from build123d import *

# Parameters (mm, degrees)
F0_R     = 25.4
F1_DEPTH = 12.7
F2_R     = 8.6995
F3_DEPTH = 25.4
F4_W     = 19.947653
F4_H     = 8.920466
F5_DEPTH = 6.35
F6_SIZE  = 0.635


with BuildPart() as f1:
    # F0 (on Top) → F1 (new body)
    with BuildSketch(Plane.XY):
        Circle(F0_R)
    extrude(amount=F1_DEPTH)

    # F2 (on face) → F3 (cut)
    with BuildSketch(Plane.XY.offset(12.7)):
        Circle(F2_R)
    extrude(amount=-F3_DEPTH, mode=Mode.SUBTRACT)

    # F4 (on face) → F5 (cut)
    with BuildSketch(Plane.XY.offset(12.7)):
        with Locations((-17.442937, 0)):
            Rectangle(F4_W, F4_H)
    extrude(amount=-F5_DEPTH, mode=Mode.SUBTRACT)

    # F6
    f6_edges = [f1.edges().sort_by_distance(p)[0] for p in [
        (-8.6995, 0, 0),
    ]]
    chamfer(f6_edges, length=F6_SIZE)


solid = f1.part
Build history of the part. All positions in model axes, mm. A direction names the side the tool comes from. Round coordinates to 2 decimals unless told otherwise and drop trailing zeros. Write each loop counter-clockwise with the first axis right and the second up, starting at its lowest first coordinate (ties: lowest second). Pieces come first, ordered by that corner, then holes. Notation, with made-up numbers: M 77.5,14 L 130.5,14 A21 ccw 130.5,40 Z; hole C 46,21.25 d7. An arc over 180 degrees is marked long. Answer in a Markdown table with one row per item.
1. Which spindle directions (+Z, -Z, +X, -X, +Y, -Y) get a long thin tool onto all of the face, cutting with end or side? Do faces 1 (the face through (11, 0, 12.7)), 2 (the face through (-17, 0, 6.35)). Say none if no direction does.
Geometry check:
| item | result |
|---|---|
| face 1 | +Z, +X, -X, +Y, -Y |
| face 2 | +Z, -X |
2. Saw through at D-D (y = 19.5). List the corners of the cut face in (x, z).
Geometry check:
| item | result |
|---|---|
| outline | M -16.28,0 L 16.28,0 L 16.28,12.7 L -16.28,12.7 Z |
3. Probe L1, parallel to Y at x = 0, z = 9.25; L2, parallel to Y at x = -2, z = 5.75; L3, parallel to X at y = -4, z = 6. List the from-to ranges inside material, lowest first. Write a range as [from, to].
Geometry check:
| item | result |
|---|---|
| L1 | [-25.4, -8.7], [8.7, 25.4] |
| L2 | [-25.32, -8.47], [8.47, 25.32] |
| L3 | [-25.08, -7.73], [7.73, 25.08] |
4. Saw through at B-B (x = -19.5). List the corners of the cut face in (y, z).
Geometry check:
| item | result |
|---|---|
| outline | M -16.28,0 L 16.28,0 L 16.28,12.7 L 4.46,12.7 L 4.46,6.35 L -4.46,6.35 L -4.46,12.7 L -16.28,12.7 Z |
5. Saw through at A-A (x = 0). List the corners of the cut face in (y, z) (1 decimal).
Geometry check:
| item | result |
|---|---|
| outline | M -25.4,0 L -9.3,0 L -8.7,0.6 L -8.7,12.7 L -25.4,12.7 Z; M 8.7,0.6 L 9.3,0 L 25.4,0 L 25.4,12.7 L 8.7,12.7 Z |
6. Mould opens along X. For faces 3 (the face through (-16, 4.46, 10)), 4 (the face through (8.3, 2.6, 6.8)), 5 (the face through (24.227, 7.629, 6.261)) say: +X half, -X half, draft (parallel to the pull), parting line (faces both ways), or undercut.
Geometry check:
| item | result |
|---|---|
| face 3 | draft |
| face 4 | undercut |
| face 5 | parting line |
7. Saw through at C-C (z = 7.25). List the corners of the cut face in (x, y), and give its area (3 significant figures).
Geometry check:
| item | result |
|---|---|
| outline | M -25.01,-4.46 A25.4 ccw long -25.01,4.46 L -7.47,4.46 A8.7 cw long -7.47,-4.46 Z |
| area | 1,640 mm2 |
8. Flat gauge pins, fed straight in: P1, Ø1, axis at x = 8.5, z = 6, coming from the -Y side; P2, Ø3, axis at x = -13, z = 8.5, coming from the -Y side; P3, Ø2.5, axis at x = -17, y = -2, coming from the +Z side. Where does each tip first touch, or does it go through?
Geometry check:
| item | result |
|---|---|
| P1 | y = -24.11 |
| P2 | y = -22.65 |
| P3 | z = 6.35 |
